Drawing for the job (mm, zero at the part's lowest x, y, z). Round coordinates to 2 decimals unless told otherwise and drop trailing zeros. Loops run counter-clockwise (first coordinate to the right, second up) from the corner with the lowest first, then second, coordinate; pieces in that order, holes last.
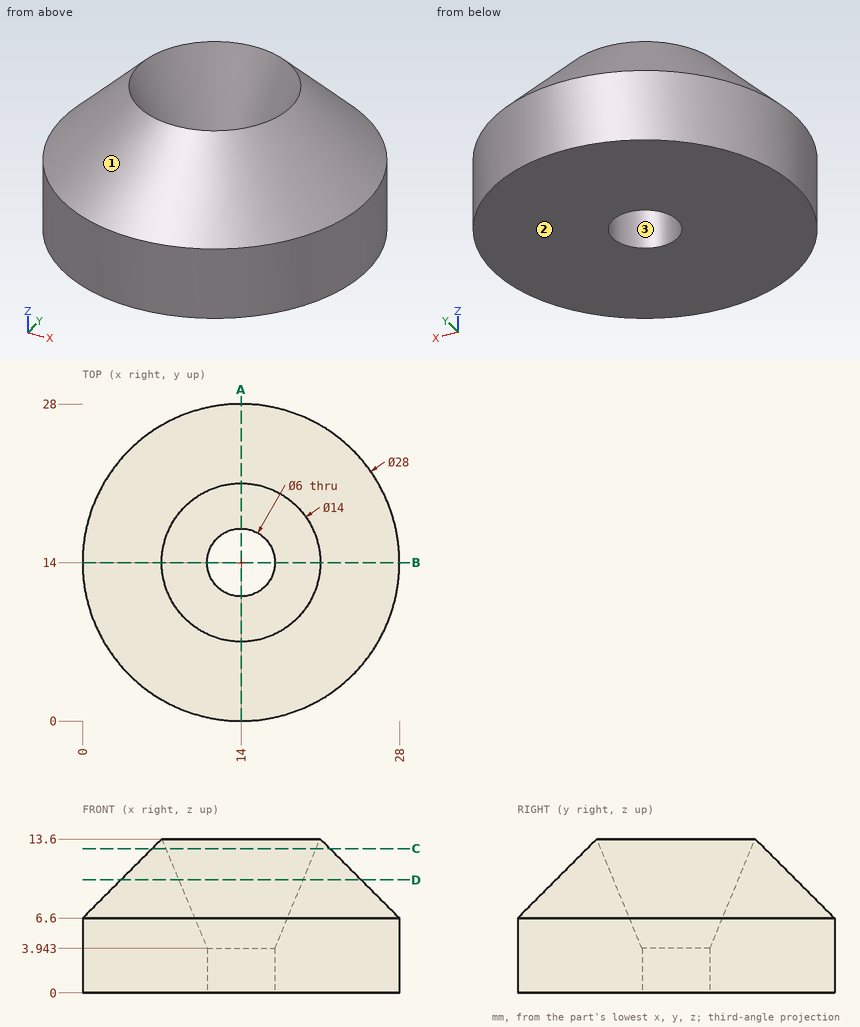
Q1. Probe line 1 (Y direction, x = 14, z = 2.15); line 2 (X direction, y = 18, z = 11.5) (1 decimal); line 3 (Z direction, x = 7.25, y = 26). List the from-to ranges inside material, lowest first.
Q2. Slice it at A-A on x = 14. Give the cut face in (y, z).
Q3. Slice it at C-C on z = 12.75. Give the cut face in (x, y).
Q4. Flat gauge pins, fed straight in: P1, Ø1.5, axis at x = 11, z = 9.5, coming from the +Y side; P2, Ø1.5, axis at x = 19.5, z = 1.5, coming from the +Y side; P3, Ø12, axis at x = 6.5, y = 10.5, coming from the -Z side; P4, Ø5, axis at x = 24.5, z = 8, coming from the +Y side. Where does each tip first touch, or does it go through?
Q5. Pull direction X, two halves, no side cores. Call the marked faces 1, 2 and 3: pulls with the +X half, pulls with the -X half, needs draft (parallel to the pull), parting line crosses it, or undercut.
Q6. Slice it at D-D on z = 10. Give the cut face in (x, y), plus the area to 3 significant figures.
Reply:
1. line 1: y = 0 to 11, 17 to 28
1. line 2: x = 5.8 to 9.4, 18.6 to 22.2
1. line 3: z = 0 to 6.83
2. outline: (0, 0) - (11, 0) - (11, 3.94) - (7, 13.6) - (0, 6.6) - close; (17, 0) - (28, 0) - (28, 6.6) - (21, 13.6) - (17, 3.94) - close
3. outline: circle Ø15.7 at (14, 14); hole circle Ø13.3 at (14, 14)
4. P1: stops at y = 25.49
4. P2: stops at y = 27.17
4. P3: stops at z = 0
4. P4: stops at y = 25.18
5. face 1: parting line crosses it
5. face 2: needs draft
5. face 3: undercut
6. outline: circle Ø21.2 at (14, 14); hole circle Ø11.02 at (14, 14)
6. area: 258 mm2
